from build123d import *

# Parameters (mm, degrees)
SKETCH2_W                    = 122.936
SKETCH2_H                    = 76.2
BOSS_EXTRUDE1_DEPTH          = 3.175
F_10_0_1935_DIAMETER_HOLE1_D = 4.9784
LPATTERN1_COUNT              = 2
LPATTERN1_PITCH              = 60.452
F_1_4_0_25_DIAMETER_HOLE1_D  = 6.7564
MIRROR1_COPY_1_D             = 4.9784
SKETCH7_R                    = 12.7
CUT_EXTRUDE1_DEPTH           = 4.175


with BuildPart() as part:
    # Sketch2 → Boss-Extrude1 (new body)
    with BuildSketch(Plane(origin=(0, 0, 0), x_dir=(1, 0, 0), z_dir=(0, 1, 0))):
        with Locations((61.468, 38.1)):
            Rectangle(SKETCH2_W, SKETCH2_H)
    extrude(amount=BOSS_EXTRUDE1_DEPTH)

    # #10 (0.1935) Diameter Hole1 (through all)
    with Locations(Plane(origin=(0, 3.175, 0), x_dir=(1, 0, 0), z_dir=(0, 1, 0))):
        with Locations((4.826, 69.85)):
            f_10_0_1935_diameter_hole1 = Hole(F_10_0_1935_DIAMETER_HOLE1_D / 2)

    # LPattern1: #10 (0.1935) Diameter Hole1 ×2
    with Locations(*[(i * LPATTERN1_PITCH, 0, 0) for i in range(1, LPATTERN1_COUNT)]):
        add(f_10_0_1935_diameter_hole1, mode=Mode.SUBTRACT)

    # 1/4 (0.25) Diameter Hole1 (through all)
    with Locations(Plane(origin=(0, 3.175, 0), x_dir=(1, 0, 0), z_dir=(0, 1, 0))):
        with Locations((110.236, 63.5)):
            f_1_4_0_25_diameter_hole1 = Hole(F_1_4_0_25_DIAMETER_HOLE1_D / 2)

    # Mirror1: 1/4 (0.25) Diameter Hole1, #10 (0.1935) Diameter Hole1 across plane
    add(f_1_4_0_25_diameter_hole1.mirror(Plane(origin=(0, 0, -38.1), x_dir=(1, 0, 0), z_dir=(0, 0, -1))), mode=Mode.SUBTRACT)
    add(f_10_0_1935_diameter_hole1.mirror(Plane(origin=(0, 0, -38.1), x_dir=(1, 0, 0), z_dir=(0, 0, -1))), mode=Mode.SUBTRACT)

    # Mirror1 copy 1 (through all)
    with Locations(Plane(origin=(60.452, 3.175, -76.2), x_dir=(1, 0, 0), z_dir=(0, 1, 0))):
        with Locations((4.826, -69.85)):
            Hole(MIRROR1_COPY_1_D / 2)

    # Sketch7 → Cut-Extrude1 (cut, through all)
    with BuildSketch(Plane(origin=(0, 3.175, 0), x_dir=(1, 0, 0), z_dir=(0, 1, 0))):
        with Locations((35.052, 16.764)):
            Circle(SKETCH7_R)
        with Locations((35.052, 52.324)):
            Circle(SKETCH7_R)
    extrude(amount=-CUT_EXTRUDE1_DEPTH, mode=Mode.SUBTRACT)


solid = part.part
Model file for the job. Use its own axes, mm. Coordinates: 2 decimals unless noted, no trailing zeros. Write each loop counter-clockwise with the first axis right and the second up, starting at its lowest first coordinate (ties: lowest second). Pieces come first, ordered by that corner, then holes. Notation, with made-up numbers: (74, -11.5) - (108, -11.5) arc R23 cw to (108, 1.5) - close; hole circle Ø10 at (-7, -12.5). An arc over 180 degrees is marked (long way). Write each question's results on one line, items separated by ' | '. Start each with the question number.
1) Probe line 1 along X through (y, z) = (1.85, -69.85); line 2 along X through (y, z) = (0.25, -68.5); line 3 along X through (y, z) = (2.2, -6.35). List the from-to ranges inside material, lowest first. Write a range as from..to.
2) Cut at C-C (x = 34). Write the cut outline in (y, z) (3 decimals), then the cut area to 3 significant figures.
3) Cut at D-D (y = 2.3). Count the separate pieces of the cut face and the enclosed holes in it, then the cut area to 3 significant figures.
4) Mould opens along Z. For faces 1 (the face through (3.49, 1.57, -4.25)), 2 (the face through (122.936, 2, -38)), 3 (the face through (67.765, 1.565, -6.459)), 4 (the face through (61, 2, 0)) say: pulls with the +Z half, pulls with the -Z half, needs draft (parallel to the pull), parting line crosses it, or undercut.
5) Cut at A-A (z = -69.85). Write the cut outline in (x, y) (3 decimals).
6) Cut at B-B (z = -6.35). Write the cut outline in (x, y) (3 decimals).
7) Flat gauge pins, fed straight in: P1, Ø6, axis at x = 110.236, z = -63.5, coming from the -Y side; P2, Ø6.5, axis at x = 4.826, z = -6.35, coming from the -Y side. Where does each tip first touch, or does it go through?
Returned:
1) line 1: 0..2.34, 7.32..62.79, 67.77..122.94 | line 2: 0..2.73, 6.92..63.19, 67.37..122.94 | line 3: 0..2.34, 7.32..27.78, 42.32..62.79, 67.77..122.94
2) outline: (0, -76.2) - (3.175, -76.2) - (3.175, -64.98) - (0, -64.98) - close; (0, -39.668) - (3.175, -39.668) - (3.175, -29.42) - (0, -29.42) - close; (0, -4.108) - (3.175, -4.108) - (3.175, 0) - (0, 0) - close | area: 81.2 mm^2
3) separate pieces: 1 | enclosed holes: 8 | area: 8,200 mm^2
4) face 1: undercut | face 2: needs draft | face 3: undercut | face 4: pulls with the +Z half
5) outline: (0, 0) - (2.337, 0) - (2.337, 3.175) - (0, 3.175) - close; (7.315, 0) - (62.789, 0) - (62.789, 3.175) - (7.315, 3.175) - close; (67.767, 0) - (122.936, 0) - (122.936, 3.175) - (67.767, 3.175) - close
6) outline: (0, 0) - (2.337, 0) - (2.337, 3.175) - (0, 3.175) - close; (7.315, 0) - (27.783, 0) - (27.783, 3.175) - (7.315, 3.175) - close; (42.321, 0) - (62.789, 0) - (62.789, 3.175) - (42.321, 3.175) - close; (67.767, 0) - (122.936, 0) - (122.936, 3.175) - (67.767, 3.175) - close
7) P1: through | P2: y = 0
